Model file for the job. Use its own axes, mm. A direction names the side the tool comes from. Give positions to 0.01 mm unless a question says otherwise; leave off trailing zeros. Order: outer loops, then holes, each group sorted by start corner. A loop starts at its lowest first (then second) coordinate and runs counter-clockwise, first axis right, second up. Notation, with made-up numbers: M 58,83 L 72,83 A30 ccw 72,113 Z; hole C 24,6.5 d5. An arc over 180 degrees is marked long. Return JSON: item names as keys, results as strings. Group by question number.
1. Two-plate mould, pull along Y, no slides. Class faces 1 (the face through (-15, 45.2, 1.5)), 2 (the face through (-0.08, 38.75, 8.95)), 3 (the face through (8.2, 0, -1.5)): released by +Y, released by -Y, zero draft, split by the parting line, or undercut.
2. Pin check, flat tips, straight feed: pin 1 (4 mm diameter, centred on x = 0, y = 10, fed in from -Z); pin 2 (10 mm diameter, centred on y = 15.5, z = -1.5, fed in from +X); pin 3 (3 mm diameter, centred on y = 6, z = 7.5, fed in from -X); pin 4 (6 mm diameter, centred on x = -2.5, z = -7, fed in from +Y). Stop position of each tip, or through.
3. Slice it at A-A on z = 0. List the corners of the cut face in (x, y) (3 decimals).
4. Slice it at C-C on y = 43. List the corners of the cut face in (x, z), then the cut area to 3 significant figures.
5. Slice it at D-D on x = 12. List the corners of the cut face in (y, z) (3 decimals), then the cut area to 3 significant figures.
6. Wall check: probe 1 along Z at (x, y) = (0, 7) (3 decimals); probe 2 along X at (y, z) = (37, -8.5); probe 3 along Y at (x, z) = (0, 8.7). Give the ranges that are in metal, low to high. Write a range as [from, to].
7. 3-axis set-ups, long thin cutter, end or side, ignore diameter. For faces 4 (the face through (-1.75, 10.08, -8.98)), 5 (the face through (0.21, 46.915, 1.302)), 6 (the face through (8.43, 13.66, 5.38)): which of +Z, -Z, +X, -X, +Y, -Y reach the whole face in a straight line?
8. Slice it at B-B on y = 37. List the corners of the cut face in (x, z) (3 decimals), then the cut area to 3 significant figures.
from build123d import *

# Parameters (mm, degrees)
SKETCH1_R                = 10
SKETCH1_R_2              = 8.125
BOSS_EXTRUDE1_DEPTH      = 25
SKETCH2_R                = 10
SKETCH2_R_2              = 8.125
BOSS_EXTRUDE2_DEPTH      = 15
BOSS_EXTRUDE4_REACH      = 32.822
BOSS_EXTRUDE4_END_RADIUS = 10
SKETCH4_R                = 10
CUT_EXTRUDE3_REACH       = 32.822
SKETCH7_R                = 8.125
CUT_EXTRUDE1_DEPTH       = 51.338851795
CUT_EXTRUDE1_DEPTH_BACK  = 51.338851795
SKETCH5_R                = 1.75
CUT_EXTRUDE2_DEPTH       = 51.338851814
CUT_EXTRUDE2_DEPTH_BACK  = 51.338851814
SKETCH6_R                = 1.75


with BuildPart() as part:
    # Sketch1 → Boss-Extrude1 (new body)
    with BuildSketch(Plane(origin=(0, 0, 0), x_dir=(1, 0, 0), z_dir=(0, 1, 0))):
        with Locations(Location((0, 0, 0), (0, 0, 270))):
            Circle(SKETCH1_R)
        with Locations(Location((0, 0, 0), (0, 0, 270))):
            Circle(SKETCH1_R_2, mode=Mode.SUBTRACT)
    extrude(amount=BOSS_EXTRUDE1_DEPTH)



with BuildPart() as body_2:
    # Sketch2 → Boss-Extrude2 (new, symmetric)
    with BuildSketch(Plane(origin=(0, 0, 0), x_dir=(0, 0, -1), z_dir=(1, 0, 0))):
        with Locations((0, 37)):
            Circle(SKETCH2_R)
        with Locations((0, 37)):
            Circle(SKETCH2_R_2, mode=Mode.SUBTRACT)
    extrude(amount=BOSS_EXTRUDE2_DEPTH, both=True)


with BuildPart() as part_1:
    add(part.part)

    add(body_2.part)  # Boss-Extrude4 merges body 2
    # Boss-Extrude4: up to this cylinder (the profile starts outside it)
    boss_extrude4_end = Plane(origin=(0, 37, 0), z_dir=(-1, 0, 0)) * Cylinder(BOSS_EXTRUDE4_END_RADIUS, 86.644, mode=Mode.PRIVATE)
    # Sketch4 → Boss-Extrude4 (add, up to the surface)
    with BuildSketch(Plane(origin=(0, 25, 0), x_dir=(1, 0, 0), z_dir=(0, 1, 0)), mode=Mode.PRIVATE) as boss_extrude4_sk1:
        with Locations(Location((0, 0, 0), (0, 0, 270))):
            Circle(SKETCH4_R)
    boss_extrude4_tool1 = extrude(boss_extrude4_sk1.sketch, amount=BOSS_EXTRUDE4_REACH, mode=Mode.PRIVATE) - boss_extrude4_end
    add(boss_extrude4_tool1.solids().sort_by_distance((0, 25, 0))[0])

    # Sketch7 → Cut-Extrude3 (cut, up to next)
    with BuildSketch(Plane.XZ.offset(-25), mode=Mode.PRIVATE) as cut_extrude3_sk1:
        with Locations(Location((0, 0, 0), (0, 0, 90))):
            Circle(SKETCH7_R)
    cut_extrude3_tool1 = extrude(cut_extrude3_sk1.sketch, amount=-CUT_EXTRUDE3_REACH, mode=Mode.PRIVATE) & part_1.part
    add(cut_extrude3_tool1.solids().sort_by_distance((0, 25, 0))[0], mode=Mode.SUBTRACT)

    # Sketch5 → Cut-Extrude1 (cut, two sides: drawn at the far end of the back side and taken through both)
    with BuildSketch(Plane.XY.offset(-CUT_EXTRUDE1_DEPTH_BACK)):
        with Locations((0, 10)):
            Circle(SKETCH5_R)
    extrude(amount=CUT_EXTRUDE1_DEPTH + CUT_EXTRUDE1_DEPTH_BACK, mode=Mode.SUBTRACT)

    # Sketch6 → Cut-Extrude2 (cut, two sides: drawn at the far end of the back side and taken through both)
    with BuildSketch(Plane.XY.offset(-CUT_EXTRUDE2_DEPTH_BACK)):
        with Locations(Location((0, 37, 0), (0, 0, 314.999999393))):
            Circle(SKETCH6_R)
    extrude(amount=CUT_EXTRUDE2_DEPTH + CUT_EXTRUDE2_DEPTH_BACK, mode=Mode.SUBTRACT)


solid = part_1.part
Result:
{
 "1": {"face 1": "zero draft", "face 2": "undercut", "face 3": "released by -Y"},
 "2": {"pin 1": "stops at z = -10", "pin 2": "stops at x = 10", "pin 3": "stops at x = -8", "pin 4": "stops at y = 46.17"},
 "3": {"outline": "M -15,27 L -10,27 L -10,0 L -8.125,0 L -8.125,28.875 L -15,28.875 Z; M -15,45.125 L 15,45.125 L 15,47 L -15,47 Z; M 8.125,0 L 10,0 L 10,27 L 15,27 L 15,28.875 L 8.125,28.875 Z"},
 "4": {"outline": "M -15,-8 L 15,-8 L 15,-5.48 L -15,-5.48 Z; M -15,5.48 L 15,5.48 L 15,8 L -15,8 Z", "area": "151 mm2"},
 "5": {"outline": "C 37,0 d20; hole C 37,0 d16.25", "area": "107 mm2"},
 "6": {"probe 1": "z = [-10, -8.125], [8.125, 10]", "probe 2": "x = [-15, -1.75], [1.75, 15]", "probe 3": "y = [0, 8.25], [11.75, 35.25], [38.75, 41.93]"},
 "7": {"face 4": "+Z, -Z", "face 5": "none", "face 6": "-Y"},
 "8": {"outline": "M -15,-10 L -1.75,-10 L -1.75,-8.125 L -15,-8.125 Z; M -15,8.125 L -1.75,8.125 L -1.75,10 L -15,10 Z; M 1.75,-10 L 15,-10 L 15,-8.125 L 1.75,-8.125 Z; M 1.75,8.125 L 15,8.125 L 15,10 L 1.75,10 Z", "area": "99.4 mm2"}
}
